Check sheet for the modelled part. Datum: model origin and axes. Units: mm. Round coordinates to 2 decimals unless told otherwise and drop trailing zeros. Loops run counter-clockwise (first coordinate to the right, second up) from the corner with the lowest first, then second, coordinate; pieces in that order, holes last. Notation, with made-up numbers: M -4.75,85.5 L 31.25,85.5 A31 cw 31.25,113.5 Z; hole C -8.75,28 d10. An arc over 180 degrees is marked long. One line per question, with ' | ' between items. Start each with the question number.
(1) Section check A-A (x = 0). Record the boundary of the cut face in (y, z), and give its area (3 significant figures).
(2) Section check B-B (y = 10.5). Record the boundary of the cut face in (x, z), and give its area (3 significant figures).
(3) Section check C-C (z = 326). Record the boundary of the cut face in (x, y), and give its area (3 significant figures).
(4) Go/stop test with flat-tipped pins: P1, Ø19, axis at x = -3.5, z = 24, coming from the +Y side; P2, Ø1.5, axis at x = -13.5, z = 164.5, coming from the +Y side; P3, Ø4.5, axis at x = 19, z = 179, coming from the -Y side; P4, Ø4, axis at x = -9.5, y = 12, coming from the -Z side. Record where each tip stops, or that it passes through.
(5) Thickness scan on probe 1 along Y at (x, z) = (0, 140); probe 2 along X at (y, z) = (8.5, 309); probe 3 along X at (y, z) = (16, 59). Record the ranges inside material, lowest first. Write a range as [from, to].
Autodesk Inventor part; units mm, degrees
ref_plane "Work Plane1" through (0, 0, 32) normal (0, 0, 1) x (1, 0, 0)
ref_plane "YZ Plane" through (0, 0, 0) normal (1, 0, 0) x (0, 1, 0)
ref_plane "XZ Plane" through (0, 0, 0) normal (0, 1, 0) x (-1, 0, 0)
sketch "Sketch1" plane through (0, 0, 0) normal (0, 0, 1) x (1, 0, 0)
  circle A0 centre (0, 0) radius 21.08
  circle A1 centre (0, 0) radius 17.35
  dimension "d0" = 42.16
  dimension "d1" = 3.73
extrude "Extrusion1" add sketch "Sketch1" along normal blind 445
ref_plane "Work Plane1" through (0, 0, 32) normal (0, 0, 1) x (1, 0, 0)
sketch "Sketch6" plane through (0, 0, 32) normal (0, 0, 1) x (1, 0, 0)
  line L0 (11.1371, -22.214) -> (-11.1371, -22.214)
  line L1 (-11.1371, -22.214) -> (-11.1371, -18)
  line L2 (-11.1371, -18) -> (11.1371, -18)
  line L3 (11.1371, -18) -> (11.1371, -22.214)
  line L4 (0, -22.214) -> (0, -18) construction
  line L5 (0, 0) -> (0, -21.08) construction
  circle A0 centre (0, 0) radius 21.08
  line L6 (0, 0) -> (6.3886, 0) construction
  line L7 (11.1371, 22.214) -> (-11.1371, 22.214)
  line L8 (-11.1371, 22.214) -> (-11.1371, 18)
  line L9 (-11.1371, 18) -> (11.1371, 18)
  line L10 (11.1371, 18) -> (11.1371, 22.214)
  line L11 (0, 22.214) -> (0, 18) construction
  point P0 (20.2483, 5.8629)
  point P1 (21.08, 0)
  point P2 (0, 21.08)
  dimension "d10" = 18
extrude "Extrusion4" cut sketch "Sketch6" against normal blind 17.5 contours L0 L1 L2 A0 L3 | A0 L2 | L9 L8 L7 L10 A0 | A0 L9
sketch "Sketch7" plane through (0, 0, 445) normal (0, 0, 1) x (1, 0, 0)
  line L0 (30, -5.75) -> (0, -5.75)
  line L1 (0, -5.75) -> (0, 5.75)
  line L2 (0, 5.75) -> (30, 5.75)
  line L3 (30, 5.75) -> (30, -5.75)
  point P0 (0, 0)
  point P1 (0, 0)
  dimension "d13" = 30
  dimension "d14" = 11.5
extrude "Extrusion5" cut sketch "Sketch7" against normal up to next
properties part number "outer_sheath" material "Acetal Resin, White"
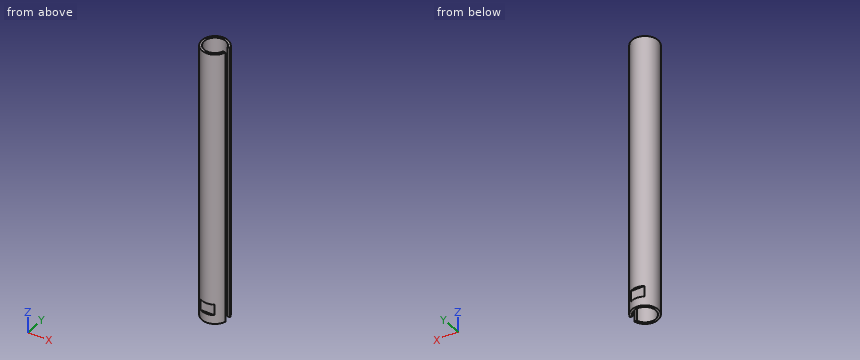
The answers:
1) outline: M -21.08,0 L -17.35,0 L -17.35,445 L -21.08,445 L -21.08,32 L -18,32 L -18,14.5 L -21.08,14.5 Z; M 17.35,0 L 21.08,0 L 21.08,14.5 L 18,14.5 L 18,32 L 21.08,32 L 21.08,445 L 17.35,445 Z | area: 3,210 mm²
2) outline: M -18.28,0 L -13.81,0 L -13.81,445 L -18.28,445 Z; M 13.81,0 L 18.28,0 L 18.28,445 L 13.81,445 Z | area: 3,980 mm²
3) outline: M 16.37,-5.75 A17.35 cw long 16.37,5.75 L 20.28,5.75 A21.08 ccw long 20.28,-5.75 Z | area: 407 mm²
4) P1: y = 21.08 | P2: y = 16.79 | P3: y = -12.8 | P4: through
5) probe 1: [-21.08, -17.35], [17.35, 21.08] | probe 2: [-19.29, -15.13], [15.13, 19.29] | probe 3: [-13.72, -6.71], [6.71, 13.72]
